Model file for the job. Use its own axes, mm. Face numbers are marked on the shaded views. A direction names the side the tool comes from. Give positions to 0.01 mm unless a question says otherwise; leave off trailing zeros. Write each loop counter-clockwise with the first axis right and the second up, starting at its lowest first coordinate (ties: lowest second). Pieces come first, ordered by that corner, then holes. Notation, with made-up numbers: (-12, 5.25) - (42, 5.25) arc R31 cw to (42, 42.25) - close; hole circle Ø5 at (78.25, 85). An arc over 180 degrees is marked (long way). Use a Markdown table: item, result. Add a question column.
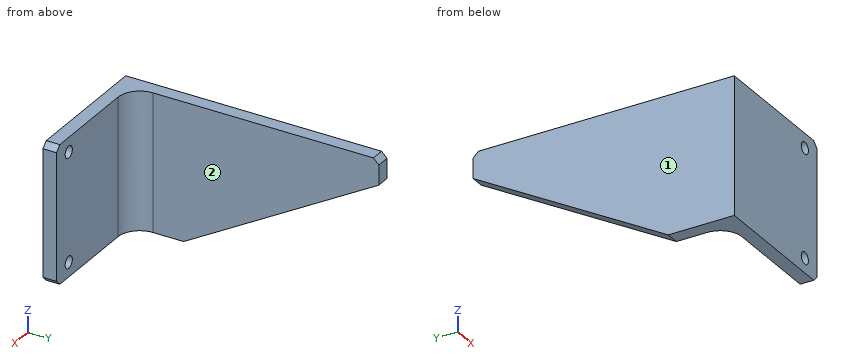
```python
from build123d import *

# Parameters (mm, degrees)
ESBO_O1_W                = 63.48
ESBO_O1_H                = 63.4
RESSALTO_EXTRUS_O1_DEPTH = 6.27
CHANFRO1_SIZE            = 2.5
RESSALTO_EXTRUS_O2_DEPTH = 6.27
CHANFRO2_SIZE            = 2.5
FILETE1_R                = 10
ESBO_O3_R                = 2.75
CORTE_EXTRUS_O1_DEPTH    = 6.27


with BuildPart() as part:
    # Esboço1 → Ressalto-extrusão1 (new body)
    with BuildSketch(Plane(origin=(0, 0, 0), x_dir=(1, 0, 0), z_dir=(0, 1, 0))):
        Rectangle(ESBO_O1_W, ESBO_O1_H)
    extrude(amount=RESSALTO_EXTRUS_O1_DEPTH)

    # Chanfro1
    chanfro1_edges = [part.edges().sort_by_distance(p)[0] for p in [
        (31.74, 3.135, -31.7),
        (31.74, 3.135, 31.7),
    ]]
    chamfer(chanfro1_edges, length=CHANFRO1_SIZE)

    # Esboço2 → Ressalto-extrusão2 (add)
    with BuildSketch(Plane.ZY.offset(25.49)):
        Polygon((-31.7, 30.5), (-31.7, 0), (31.7, 0), (31.7, 30.5), (31.7, 120.63), (20.05, 120.63), align=None)
    extrude(amount=RESSALTO_EXTRUS_O2_DEPTH)

    # Chanfro2
    chanfro2_edges = [part.edges().sort_by_distance(p)[0] for p in [
        (-28.625, 120.63, 31.7),
    ]]
    chamfer(chanfro2_edges, length=CHANFRO2_SIZE)

    # Filete1
    filete1_edges = [part.edges().sort_by_distance(p)[0] for p in [
        (-25.49, 6.27, 0),
    ]]
    fillet(filete1_edges, radius=FILETE1_R)

    # Esboço3 → Corte-extrusão1 (cut)
    with BuildSketch(Plane(origin=(0, 0, 0), x_dir=(-1, 0, 0), z_dir=(0, -1, 0))):
        with Locations((-22.39, -25)):
            Circle(ESBO_O3_R)
        with Locations((-22.39, 25)):
            Circle(ESBO_O3_R)
    extrude(amount=-CORTE_EXTRUS_O1_DEPTH, mode=Mode.SUBTRACT)


solid = part.part
```
(1) Band-saw the part on A-A (z = 25). Write the cut outline in (x, y).
(2) Probe probe 1 along Z at (x, y) = (22.39, 2.75); probe 2 along X at (y, z) = (4.25, 25); probe 3 along Y at (x, z) = (-13, 4.5). List the from-to ranges inside material, lowest first. Write a range as [from, to].
(3) Band-saw the part on B-B (x = 22.39). Write the cut outline in (y, z).
(4) Band-saw the part on C-C (y = 24.5). Write the cut outline in (x, z), then the cut area to 3 significant figures.
(5) Which spindle directions (+Z, -Z, +X, -X, +Y, -Y) get a long thin tool onto all of the face, cutting with end or side? Do the marked faces 1 and 2. Say none if no direction does.
(6) Flat gauge pins, fed straight in: pin 1 (3 mm diameter, centred on x = 10, z = -20, fed in from +Y); pin 2 (3 mm diameter, centred on y = 41.5, z = -2, fed in from +X); pin 3 (10 mm diameter, centred on y = 15, z = 22.5, fed in from +X). Where does each tip first touch, or does it go through?
(7) Band-saw the part on D-D (z = -9). Write the cut outline in (x, y), then the cut area to 3 significant figures.
Model answer:
| question | item | result |
|---|---|---|
| 1 | outline | (-31.76, 0) - (19.64, 0) - (19.64, 6.27) - (-15.49, 6.27) arc R10 cw to (-25.49, 16.27) - (-25.49, 120.63) - (-31.76, 120.63) - close; (25.14, 0) - (31.74, 0) - (31.74, 6.27) - (25.14, 6.27) - close |
| 2 | probe 1 | z = [-31.7, -27.75], [-22.25, 22.25], [27.75, 31.7] |
| 2 | probe 2 | x = [-31.76, 19.64], [25.14, 31.74] |
| 2 | probe 3 | y = [0, 6.27] |
| 3 | outline | (0, -31.7) - (6.27, -31.7) - (6.27, -27.75) - (0, -27.75) - close; (0, -22.25) - (6.27, -22.25) - (6.27, 22.25) - (0, 22.25) - close; (0, 27.75) - (6.27, 27.75) - (6.27, 31.7) - (0, 31.7) - close |
| 4 | outline | (-31.76, -31.7) - (-25.49, -31.7) - (-25.49, 31.7) - (-31.76, 31.7) - close |
| 4 | area | 398 mm^2 |
| 5 | face 1 | +Z, -Z, -X, +Y, -Y |
| 5 | face 2 | +Z, -Z, +X, +Y |
| 6 | pin 1 | stops at y = 6.27 |
| 6 | pin 2 | stops at x = -25.49 |
| 6 | pin 3 | stops at x = -23.28 |
| 7 | outline | (-31.76, 0) - (31.74, 0) - (31.74, 6.27) - (-15.49, 6.27) arc R10 cw to (-25.49, 16.27) - (-25.49, 70.04) - (-31.76, 70.04) - close |
| 7 | area | 819 mm^2 |
